from build123d import *

# Parameters (mm, degrees)
SKETCH1_R           = 6
SKETCH1_R_2         = 5
BOSS_EXTRUDE1_DEPTH = 12
BOSS_EXTRUDE2_DEPTH = 12
CUT_EXTRUDE1_DEPTH  = 150.263087319


with BuildPart() as part:
    # Sketch1 → Boss-Extrude1 (new body)
    with BuildSketch(Plane(origin=(0, 0, 0), x_dir=(1, 0, 0), z_dir=(0, 1, 0))):
        with BuildLine():
            Line((-49.533874762, 40.242629587), (-113.533874762, 40.242629587))
            Line((-113.533874762, 40.242629587), (-113.533874762, 30.681729378))
            ThreePointArc((-113.533874762, 30.681729378), (-116.46280695, 23.610661566), (-123.533874762, 20.681729378))
            Line((-123.533874762, 20.681729378), (-163.533874762, 20.681729378))
            ThreePointArc((-163.533874762, 20.681729378), (-183.533874762, 0.681729378), (-163.533874762, -19.318270622))
            Line((-163.533874762, -19.318270622), (-123.533874762, -19.318270622))
            ThreePointArc((-123.533874762, -19.318270622), (-116.46280695, -22.24720281), (-113.533874762, -29.318270622))
            Line((-113.533874762, -29.318270622), (-113.533874762, -34.757370413))
            Line((-113.533874762, -34.757370413), (-49.533874762, -34.757370413))
            Line((-49.533874762, -34.757370413), (-49.533874762, 40.242629587))
        make_face()
        with Locations(Location((-163.533874762, 0.681729378, 0), (0, 0, 270))):
            Circle(SKETCH1_R, mode=Mode.SUBTRACT)
        with Locations(Location((-81.533874762, -19.257370413, 0), (0, 0, 270))):
            Circle(SKETCH1_R_2, mode=Mode.SUBTRACT)
        with Locations(Location((-81.533874762, 24.742629587, 0), (0, 0, 270))):
            Circle(SKETCH1_R_2, mode=Mode.SUBTRACT)
    extrude(amount=BOSS_EXTRUDE1_DEPTH)

    # Sketch3 → Boss-Extrude2 (add)
    with BuildSketch(Plane(origin=(-49.533874762, 0, 0), x_dir=(0, 0, -1), z_dir=(1, 0, 0))):
        with BuildLine():
            Line((-34.757370413, 12), (40.199591679, 12))
            Line((40.199591679, 12), (40.199591679, 45))
            ThreePointArc((40.199591679, 45), (38.149339148, 49.949747468), (33.199591679, 52))
            Line((33.199591679, 52), (-27.757370413, 52))
            ThreePointArc((-27.757370413, 52), (-32.707117881, 49.949747468), (-34.757370413, 45))
            Line((-34.757370413, 45), (-34.757370413, 12))
        make_face()
    boss_extrude2 = extrude(amount=-BOSS_EXTRUDE2_DEPTH)

    # Sketch5 → Cut-Extrude1 (cut, through all)
    with BuildSketch(Plane(origin=(-49.533874762, 0, 0), x_dir=(0, 0, -1), z_dir=(1, 0, 0))):
        with BuildLine():
            Line((-21.757370413, 45), (27.199591679, 45))
            ThreePointArc((27.199591679, 45), (33.199591679, 39), (27.199591679, 33))
            Line((27.199591679, 33), (-21.757370413, 33))
            ThreePointArc((-21.757370413, 33), (-27.757370413, 39), (-21.757370413, 45))
        make_face()
    cut_extrude1 = extrude(amount=-CUT_EXTRUDE1_DEPTH, mode=Mode.SUBTRACT)

    # Mirror1: Boss-Extrude2, Cut-Extrude1 across plane
    add(boss_extrude2.mirror(Plane(origin=(-81.533874762, 0, 0), x_dir=(0, 0, 1), z_dir=(1, 0, 0))))
    add(cut_extrude1.mirror(Plane(origin=(-81.533874762, 0, 0), x_dir=(0, 0, 1), z_dir=(1, 0, 0))), mode=Mode.SUBTRACT)


solid = part.part
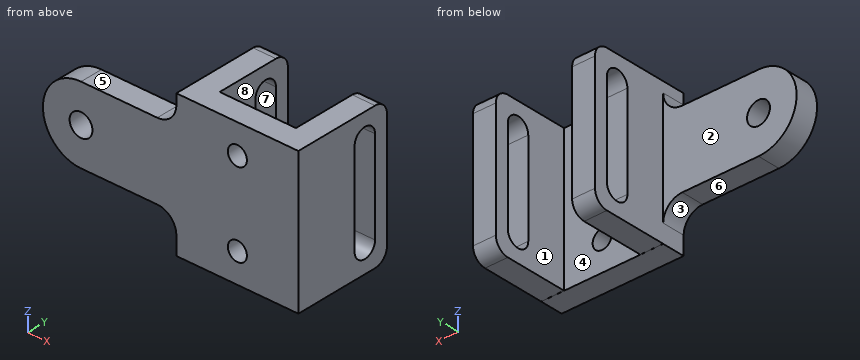
Read the model definition and answer for the solid it produces. Units are mm, in the model's axes. Face numbers are marked on the shaded views. A direction names the side the tool comes from. Coordinates: 2 decimals unless noted, no trailing zeros. Loops run counter-clockwise (first coordinate to the right, second up) from the corner with the lowest first, then second, coordinate; pieces in that order, holes last.
Q1. The part is cut by section D-D on z = -14. Write down the section's boundary in (x, y).
Q2. Each of these flat-tipped pins is pushed along its axis until it touches: pin 1 Ø6 at (x, y) = (-135, 8) entering from +Z; pin 2 Ø20 at (y, z) = (36, 6.5) entering from -X; pin 3 Ø9.5 at (x, y) = (-56, 27) entering from -Z. Where does it stop, or does it pass through?
Q3. The mould has two halves that part along X. Classify the marked faces 1, 2, 3 and 4: +X half, -X half, draft (parallel to the pull), parting line (faces both ways), or undercut.
Q4. The part is cut by section A-A on y = 39. Write down the section's boundary in (x, z).
Q5. Which of the six approach directions +Z, -Z, +X, -X, +Y, -Y give full straight-line access (tool end or side, diameter ignored) to the marked faces 5, 6, 7 and 8?
Q6. The part is cut by section B-B on y = 20. Write down the section's boundary in (x, z), and give its area (3 significant figures).
Q7. Consider probe 1 along X at (y, z) = (32, 28); probe 2 along Z at (x, y) = (-86, 7.5); probe 3 along Y at (x, z) = (-109.5, -15). Determine where each line is inside the solid, lowest interval first.
Q8. The part is cut by section C-C on x = -166.5. Write down the section's boundary in (y, z).
Results below:
1. outline: (-178.45, 0) - (-49.53, 0) - (-49.53, 33) - (-61.53, 33) - (-61.53, 12) - (-101.53, 12) - (-101.53, 33) - (-113.53, 33) - (-113.53, 12) - (-178.45, 12) - close; (-113.53, 45) - (-101.53, 45) - (-101.53, 52) - (-113.53, 52) - close; (-61.53, 45) - (-49.53, 45) - (-49.53, 52) - (-61.53, 52) - close
2. pin 1: stops at z = 19.32
2. pin 2: stops at x = -113.53
2. pin 3: stops at z = -40.2
3. face 1: undercut
3. face 2: draft
3. face 3: -X half
3. face 4: undercut
4. outline: (-113.53, -40.2) - (-101.53, -40.2) - (-101.53, -33.2) - (-113.53, -33.2) - close; (-113.53, 27.76) - (-101.53, 27.76) - (-101.53, 34.76) - (-113.53, 34.76) - close; (-61.53, -40.2) - (-49.53, -40.2) - (-49.53, -33.2) - (-61.53, -33.2) - close; (-61.53, 27.76) - (-49.53, 27.76) - (-49.53, 34.76) - (-61.53, 34.76) - close
5. face 5: +Z, -X, +Y, -Y
5. face 6: -Z, -X, +Y, -Y
5. face 7: +X, -X
5. face 8: +Z, -Z, +Y
6. outline: (-113.53, -40.2) - (-101.53, -40.2) - (-101.53, 34.76) - (-113.53, 34.76) - close; (-61.53, -40.2) - (-49.53, -40.2) - (-49.53, 34.76) - (-61.53, 34.76) - close
6. area: 1,800 mm2
7. probe 1: x = -113.53 to -101.53, -61.53 to -49.53
7. probe 2: z = -40.24 to -26.99, -22.49 to 17.01, 21.51 to 34.76
7. probe 3: y = 0 to 33, 45 to 52
8. outline: (0, -20.46) - (12, -20.46) - (12, -5.9) - (0, -5.9) - close; (0, 4.53) - (12, 4.53) - (12, 19.1) - (0, 19.1) - close
